from build123d import *

# Parameters (mm, degrees)
SKETCH_1_W               = 36
SKETCH_1_H               = 36
EXTRUDE_1_DEPTH          = 100
SKETCH_2_R               = 3
CUT_EXTRUDE_1_DEPTH      = 1
CUT_EXTRUDE_1_DEPTH_BACK = 41
SKETCH_3_OUTSIDE_W       = 64.978
SKETCH_3_OUTSIDE_H       = 124.978
CUT_EXTRUDE_2_DEPTH      = 1
CUT_EXTRUDE_2_DEPTH_BACK = 41
SKETCH_4_R               = 3
CUT_EXTRUDE_3_DEPTH      = 29
CUT_EXTRUDE_3_DEPTH_BACK = 3


with BuildPart() as part:
    # Эскиз1 → Бобышка-Вытянуть1 (new body)
    with BuildSketch(Plane.XY):
        with BuildLine():
            Line((-18, 20), (18, 20))
            ThreePointArc((18, 20), (19.414213562, 19.414213562), (20, 18))
            Line((20, 18), (20, -18))
            ThreePointArc((20, -18), (19.414213562, -19.414213562), (18, -20))
            Line((18, -20), (-18, -20))
            ThreePointArc((-18, -20), (-19.414213562, -19.414213562), (-20, -18))
            Line((-20, -18), (-20, 18))
            ThreePointArc((-20, 18), (-19.414213562, 19.414213562), (-18, 20))
        make_face()
        Rectangle(SKETCH_1_W, SKETCH_1_H, mode=Mode.SUBTRACT)
    extrude(amount=EXTRUDE_1_DEPTH)

    # Эскиз2 → Вырез-Вытянуть1 (cut, two sides)
    with BuildSketch(Plane(origin=(0, 20, 0), x_dir=(1, 0, 0), z_dir=(0, 1, 0))) as cut_extrude_1_sk:
        with Locations((0, -50)):
            Circle(SKETCH_2_R)
    extrude(amount=CUT_EXTRUDE_1_DEPTH, mode=Mode.SUBTRACT)
    extrude(cut_extrude_1_sk.sketch, amount=-CUT_EXTRUDE_1_DEPTH_BACK, mode=Mode.SUBTRACT)

    # Эскиз3 outside → Вырез-Вытянуть2 (cut, two sides)
    with BuildSketch(Plane(origin=(0, 20, 0), x_dir=(1, 0, 0), z_dir=(0, 1, 0))) as cut_extrude_2_sk:
        with Locations((0, -50)):
            Rectangle(SKETCH_3_OUTSIDE_W, SKETCH_3_OUTSIDE_H)
        with BuildLine():
            Line((6.746595399, -42.618709427), (-18, -20))
            Line((-18, -20), (-21.837410107, -20))
            Line((-21.837410107, -20), (-21.837410107, -80))
            Line((-21.837410107, -80), (-18, -80))
            Line((-18, -80), (6.746595399, -57.381290573))
            ThreePointArc((6.746595399, -57.381290573), (10, -50), (6.746595399, -42.618709427))
        make_face(mode=Mode.SUBTRACT)
    extrude(amount=CUT_EXTRUDE_2_DEPTH, mode=Mode.SUBTRACT)
    extrude(cut_extrude_2_sk.sketch, amount=-CUT_EXTRUDE_2_DEPTH_BACK, mode=Mode.SUBTRACT)

    # Эскиз4 → Вырез-Вытянуть3 (cut, two sides)
    with BuildSketch(Plane(origin=(-18, 0, 0), x_dir=(0, 0, -1), z_dir=(1, 0, 0))) as cut_extrude_3_sk:
        with Locations((-71.5, 0)):
            Circle(SKETCH_4_R)
        with Locations((-28.5, 0)):
            Circle(SKETCH_4_R)
    extrude(amount=CUT_EXTRUDE_3_DEPTH, mode=Mode.SUBTRACT)
    extrude(cut_extrude_3_sk.sketch, amount=-CUT_EXTRUDE_3_DEPTH_BACK, mode=Mode.SUBTRACT)


solid = part.part
Here's how the part is built. I have some questions about the finished solid (model axes, mm). A direction names the side the tool comes from. Coordinates: 2 decimals unless noted, no trailing zeros. Write each loop counter-clockwise with the first axis right and the second up, starting at its lowest first coordinate (ties: lowest second). Pieces come first, ordered by that corner, then holes.
Item 1: If I drill on line 1 (Y direction, x = -2.5, z = 54.5); line 2 (X direction, y = -12.5, z = 74); line 3 (X direction, y = -18.65, z = 50), over which ranges is the centre line in solid material (lowest first)?
Item 2: Will this pin go through, and if not, where does the flat tip stop? pin 1 (3 mm diameter, centred on y = 0, z = 35, fed in from +X).
Item 3: I want a section at A-A on y = 0. Write out the boundary of the cut face in (x, z).
Item 4: I want a section at D-D on x = -16. Write out the boundary of the cut face in (y, z).
Item 5: I want a section at C-C on z = 50. Write out the boundary of the cut face in (x, y).
Item 6: On a 3-axis mill with a long thin cutter (end or side, diameter ignored), from which of +Z, -Z, +X, -X, +Y, -Y can I reach the whole of each face in a straight line? I mean faces 1 (the flat face through (-18, 0, 50)), 2 (the flat face through (-7, -20, 50)). Say none if no direction works.
Item 7: I want a section at B-B on x = 1.5. Write out the boundary of the cut face in (y, z).
Item 8: If we mould it in two halves opening along Z, with no side actions, what happens to faces 3 (the flat face through (-7, -18, 50)), 4 (the cylindrical face through (-19, -1.8, 73.9)), 5 (the flat face through (-19, 0, 20))? For each: +Z half, -Z half, draft (parallel to the pull), parting line (faces both ways), or undercut.
Findings below:
1. line 1: y = -20 to -18, 18 to 20
1. line 2: x = -20 to -18
1. line 3: x = -19.89 to -3, 3 to 10
2. pin 1: stops at x = -18
3. outline: (-20, 20) - (-18, 20) - (-18, 25.5) - (-20, 25.5) - close; (-20, 31.5) - (-18, 31.5) - (-18, 68.5) - (-20, 68.5) - close; (-20, 74.5) - (-18, 74.5) - (-18, 80) - (-20, 80) - close
4. outline: (-20, 21.83) - (-18, 21.83) - (-18, 78.17) - (-20, 78.17) - close; (18, 21.83) - (20, 21.83) - (20, 78.17) - (18, 78.17) - close
5. outline: (-20, -18) arc R2 ccw to (-18, -20) - (-3, -20) - (-3, -18) - (-18, -18) - (-18, 18) - (-3, 18) - (-3, 20) - (-18, 20) arc R2 ccw to (-20, 18) - close; (3, -20) - (10, -20) - (10, -18) - (3, -18) - close; (3, 18) - (10, 18) - (10, 20) - (3, 20) - close
6. face 1: +Z, -Z, +X
6. face 2: +Z, -Z, +X, -X, -Y
7. outline: (-20, 37.82) - (-18, 37.82) - (-18, 47.4) - (-20, 47.4) - close; (-20, 52.6) - (-18, 52.6) - (-18, 62.18) - (-20, 62.18) - close; (18, 37.82) - (20, 37.82) - (20, 47.4) - (18, 47.4) - close; (18, 52.6) - (20, 52.6) - (20, 62.18) - (18, 62.18) - close
8. face 3: draft
8. face 4: undercut
8. face 5: -Z half
